Answer from the drawing. Dimensions are ordinates in mm from the lowest x, y and z of the part. Coordinates: 2 decimals unless noted, no trailing zeros. Write each loop counter-clockwise with the first axis right and the second up, starting at its lowest first coordinate (ties: lowest second). Pieces come first, ordered by that corner, then holes. Notation, with made-up numbers: (-33.75, 29) - (11.25, 29) arc R25 cw to (11.25, 56) - close; hole circle Ø5 at (-15.75, 69). An arc over 180 degrees is marked (long way). Use a Markdown table: item, result.
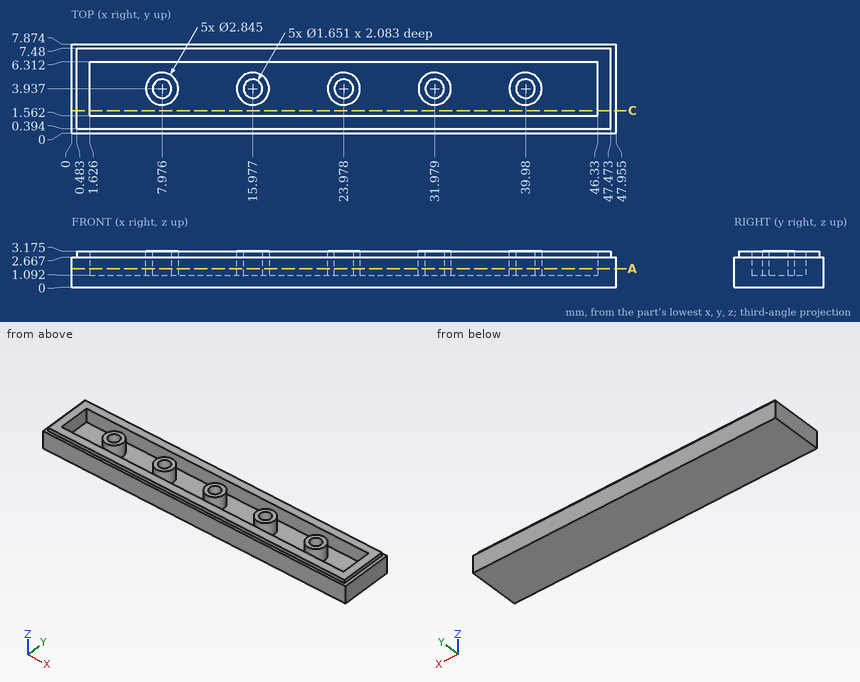
(1) Straight lines are drawn through the part: L1, parallel to Y at x = 5.5, z = 2.9; L2, parallel to Y at x = 16, z = 2.75 (1 decimal); L3, parallel to Y at x = 44, z = 1.55. For each, find the intervals that lie inside material, in ascending order.
Report:
| item | result |
|---|---|
| L1 | y = 0.39 to 1.56, 6.31 to 7.48 |
| L2 | y = 0.4 to 1.6, 2.5 to 3.1, 4.8 to 5.4, 6.3 to 7.5 |
| L3 | y = 0 to 1.56, 6.31 to 7.87 |
(2) Each of these flat-tipped pins is pushed along its axis until it touches: P1, Ø0.6, axis at x = 18, z = 3, coming from the -Y side; P2, Ø1.5, axis at x = 23.98, y = 3.94, coming from the +Z side. Where does it stop, or does it pass through?
Report:
| item | result |
|---|---|
| P1 | stops at y = 0.39 |
| P2 | stops at z = 1.09 |
(3) A cutting plane is placed at A-A, the plane z = 1.65. Count the separate pieces of the cut face and the enclosed holes in it.
Report:
| item | result |
|---|---|
| separate pieces | 6 |
| enclosed holes | 6 |
(4) A cutting plane is placed at C-C, the plane y = 2. Write down the section's boundary in (x, z) (1 decimal).
Report:
| item | result |
|---|---|
| outline | (0, 0) - (48, 0) - (48, 2.7) - (47.5, 2.7) - (47.5, 3.2) - (46.3, 3.2) - (46.3, 1.1) - (1.6, 1.1) - (1.6, 3.2) - (0.5, 3.2) - (0.5, 2.7) - (0, 2.7) - close |
